Read the model definition and answer for the solid it produces. Units are mm, in the model's axes. Face numbers are marked on the shaded views. A direction names the side the tool comes from. Coordinates: 2 decimals unless noted, no trailing zeros. Loops run counter-clockwise (first coordinate to the right, second up) from the corner with the lowest first, then second, coordinate; pieces in that order, holes last. Notation, with made-up numbers: M 60,18.25 L 117,18.25 A37 ccw 117,56.25 Z; hole C 87,67 d6. An arc over 180 degrees is marked long. One line per item, written item: value. Start each with the question number.
1. The part is cut by section D-D (z = -21). Write down the section's boundary in (x, y), then the cut area to 3 significant figures.
2. The part is cut by section A-A (y = -23). Write down the section's boundary in (x, z).
3. The part is cut by section C-C (x = 90). Write down the section's boundary in (y, z), then the cut area to 3 significant figures.
4. Consider probe 1 along X at (y, z) = (-4, 18); probe 2 along Z at (x, y) = (7.5, -10); probe 3 along Z at (x, y) = (30, -7). Determine where each line is inside the solid, lowest interval first.
5. Flat-ended cylindrical pins translate along their axes: pin 1 (1.4 mm diameter, centred on x = 37.5, z = 29, fed in from -Y); pin 2 (16.5 mm diameter, centred on x = 112.5, z = 14, fed in from -Y); pin 3 (1.5 mm diameter, centred on x = 6, z = 33, fed in from -Y). Find the tip coordinate at first contact, or state that the pin passes through.
6. The part is cut by section B-B (x = 17). Write down the section's boundary in (y, z), then the cut area to 3 significant figures.
7. For the marked faces 1 and 2, determine the directions among +Z, -Z, +X, -X, +Y, -Y from which every point of the face is accessible in a straight line to the end or side of a thin tool.
```python
from build123d import *

# Parameters (mm, degrees)
SKETCH_W               = 32
SKETCH_H               = 32
PAD_DEPTH              = 3
SKETCH001_R            = 1.45
PAD001_DEPTH           = 11
SKETCH002_W            = 15
SKETCH002_H            = 15
PAD002_DEPTH           = 7
SKETCH003_W            = 8
SKETCH003_H            = 3
PAD003_DEPTH           = 11
PAD004_DEPTH           = 3
SKETCH005_W            = 32
SKETCH005_H            = 3
PAD005_DEPTH           = 30
LINEARPATTERN_COUNT    = 4
LINEARPATTERN_PITCH    = 32
LINEARPATTERN001_COUNT = 4
LINEARPATTERN001_PITCH = 32
LINEARPATTERN002_COUNT = 4
LINEARPATTERN002_PITCH = 32
LINEARPATTERN003_COUNT = 4
LINEARPATTERN003_PITCH = 32
LINEARPATTERN004_COUNT = 4
LINEARPATTERN004_PITCH = 32
LINEARPATTERN005_COUNT = 4
LINEARPATTERN005_PITCH = 32
SKETCH006_W            = 112
SKETCH006_H            = 30
POCKET_DEPTH           = 3
PAD006_DEPTH           = 8
PAD007_DEPTH           = 8


with BuildPart() as part:
    # Sketch → Pad (new body)
    with BuildSketch(Plane.XZ):
        with Locations((16, 16)):
            Rectangle(SKETCH_W, SKETCH_H)
    pad = extrude(amount=PAD_DEPTH)

    # Sketch001 (on Face6 of Pad) → Pad001 (join)
    with BuildSketch(Plane.XZ.offset(3)):
        with Locations((6, 3)):
            Circle(SKETCH001_R)
        with Locations((26, 3)):
            Circle(SKETCH001_R)
        with Locations((26, 29)):
            Circle(SKETCH001_R)
        with Locations((6, 29)):
            Circle(SKETCH001_R)
    pad001 = extrude(amount=PAD001_DEPTH)

    # Sketch002 (on Face5 of Pad001) → Pad002 (join)
    with BuildSketch(Plane.XZ.offset(3)):
        with Locations((16, 16)):
            Rectangle(SKETCH002_W, SKETCH002_H)
    pad002 = extrude(amount=PAD002_DEPTH)

    # Sketch003 → Pad003 (join)
    with BuildSketch(Plane.XZ):
        with Locations((4, -1.5)):
            Rectangle(SKETCH003_W, SKETCH003_H)
        with Locations((4, 33.5)):
            Rectangle(SKETCH003_W, SKETCH003_H)
        with Locations((28, 33.5)):
            Rectangle(SKETCH003_W, SKETCH003_H)
        with Locations((28, -1.5)):
            Rectangle(SKETCH003_W, SKETCH003_H)
    pad003 = extrude(amount=PAD003_DEPTH)

    # Sketch004 → Pad004 (join)
    with BuildSketch(Plane.XZ):
        Polygon((0, -2.999526), (0, -27.999526), (32, -27.999526), (32, -3), (24, -3), (24, -25), (8, -25), (8, -3), align=None)
    pad004 = extrude(amount=PAD004_DEPTH)

    # Sketch005 (on Face42 of Pad004) → Pad005 (join)
    with BuildSketch(Plane.XZ.offset(3)):
        with Locations((16, -26.499526)):
            Rectangle(SKETCH005_W, SKETCH005_H)
    pad005 = extrude(amount=PAD005_DEPTH)

    # LinearPattern: Pad ×4
    with Locations(*[(i * LINEARPATTERN_PITCH, 0, 0) for i in range(1, LINEARPATTERN_COUNT)]):
        add(pad)

    # LinearPattern001: Pad001 ×4
    with Locations(*[(i * LINEARPATTERN001_PITCH, 0, 0) for i in range(1, LINEARPATTERN001_COUNT)]):
        add(pad001)

    # LinearPattern002: Pad002 ×4
    with Locations(*[(i * LINEARPATTERN002_PITCH, 0, 0) for i in range(1, LINEARPATTERN002_COUNT)]):
        add(pad002)

    # LinearPattern003: Pad003 ×4
    with Locations(*[(i * LINEARPATTERN003_PITCH, 0, 0) for i in range(1, LINEARPATTERN003_COUNT)]):
        add(pad003)

    # LinearPattern004: Pad004 ×4
    with Locations(*[(i * LINEARPATTERN004_PITCH, 0, 0) for i in range(1, LINEARPATTERN004_COUNT)]):
        add(pad004)

    # LinearPattern005: Pad005 ×4
    with Locations(*[(i * LINEARPATTERN005_PITCH, 0, 0) for i in range(1, LINEARPATTERN005_COUNT)]):
        add(pad005)

    # Sketch006 (on Face120 of LinearPattern005) → Pocket (cut)
    with BuildSketch(Plane(origin=(0, 0, -27.999526), x_dir=(1, 0, 0), z_dir=(0, 0, -1))):
        with Locations((64, 18)):
            Rectangle(SKETCH006_W, SKETCH006_H)
    extrude(amount=-POCKET_DEPTH, mode=Mode.SUBTRACT)

    # Sketch007 (on Face135 of Pocket) → Pad006 (join)
    with BuildSketch(Plane(origin=(0, 0, 0), x_dir=(0, 0, -1), z_dir=(-1, 0, 0))):
        Polygon((24.999526, 3), (18.999526, 3), (24.999526, 9), align=None)
    extrude(amount=-PAD006_DEPTH)

    # Sketch008 (on Face192 of Pad006) → Pad007 (join)
    with BuildSketch(Plane(origin=(128, 0, 0), x_dir=(0, 0, 1), z_dir=(1, 0, 0))):
        Polygon((-24.999526, 3), (-18.999526, 3), (-24.999526, 9), align=None)
    extrude(amount=-PAD007_DEPTH)


solid = part.part
```
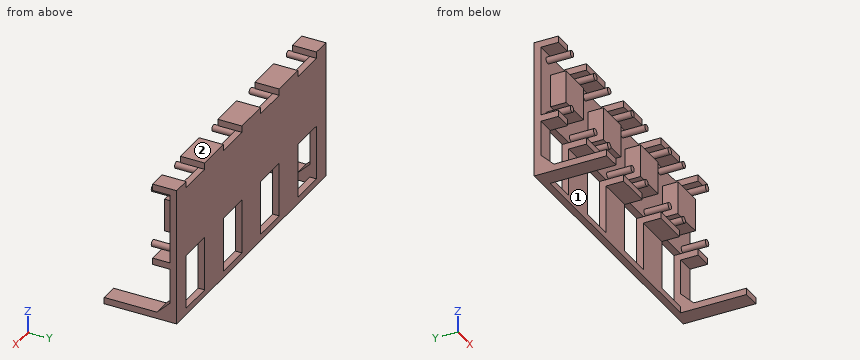
Answer block:
1. outline: M 0,-5 L 8,-5 L 8,0 L 0,0 Z; M 24,-3 L 40,-3 L 40,0 L 24,0 Z; M 56,-3 L 72,-3 L 72,0 L 56,0 Z; M 88,-3 L 104,-3 L 104,0 L 88,0 Z; M 120,-5 L 128,-5 L 128,0 L 120,0 Z
1. area: 224 mm2
2. outline: M 0,-28 L 8,-28 L 8,-25 L 0,-25 Z; M 120,-28 L 128,-28 L 128,-25 L 120,-25 Z
3. outline: M -14,1.55 L -3,1.55 L -3,0 L -11,0 L -11,-3 L -3,-3 L -3,-28 L 0,-28 L 0,35 L -11,35 L -11,32 L -3,32 L -3,30.45 L -14,30.45 L -14,27.55 L -3,27.55 L -3,4.45 L -14,4.45 Z
3. area: 301 mm2
4. probe 1: x = 8.5 to 23.5, 40.5 to 55.5, 72.5 to 87.5, 104.5 to 119.5
4. probe 2: z = -28 to -25, -3 to 0, 32 to 35
4. probe 3: z = -3 to 0, 32 to 35
5. pin 1: stops at y = -14
5. pin 2: stops at y = -10
5. pin 3: stops at y = -11
6. outline: M -10,8.5 L -3,8.5 L -3,0 L 0,0 L 0,32 L -3,32 L -3,23.5 L -10,23.5 Z; M -3,-28 L 0,-28 L 0,-25 L -3,-25 Z
6. area: 210 mm2
7. face 1: -Z, -Y
7. face 2: +Z, +X, -X, +Y, -Y
